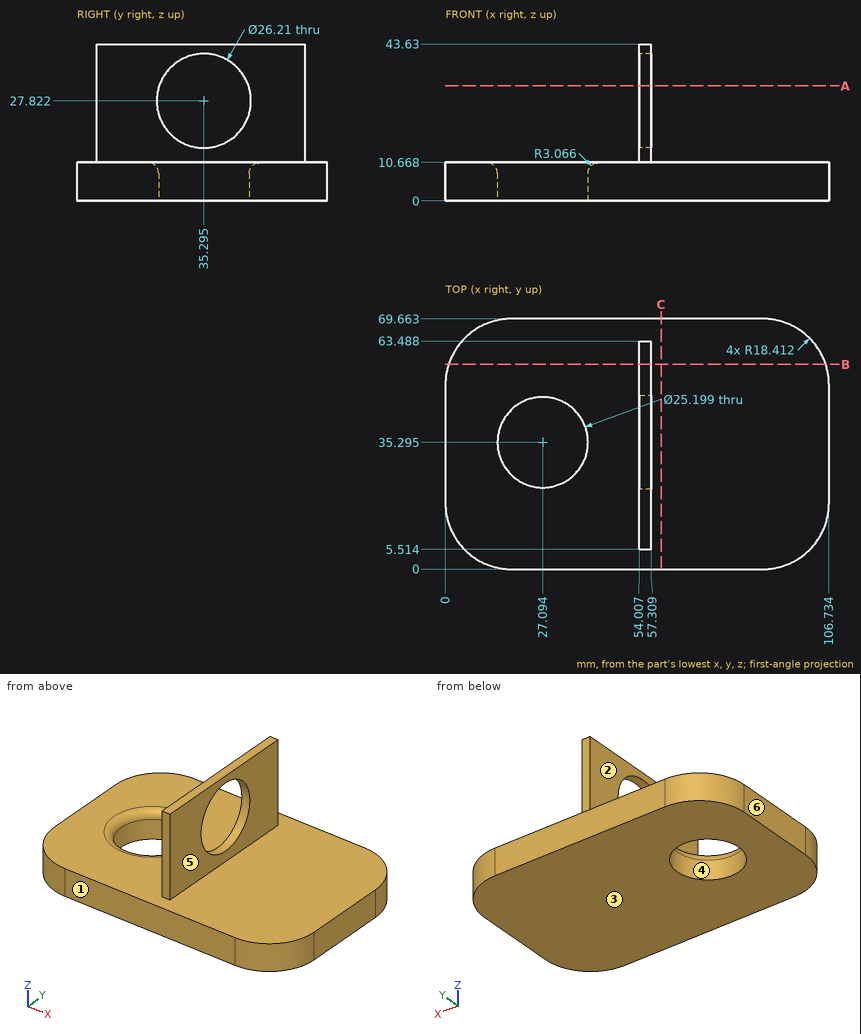
The figure shows three views and two pictorial views of one solid part (mm, origin at its lowest corner). Answer the questions. A direction names the side the tool comes from. Round coordinates to 2 decimals unless told otherwise and drop trailing zeros. Write each loop counter-clockwise with the first axis right and the second up, starting at its lowest first coordinate (ties: lowest second). Pieces come first, ordered by that corner, then holes. Notation, with made-up numbers: (-22.75, 2) - (10.25, 2) arc R17 ccw to (10.25, 20) - close; hole circle Ø2 at (21, 1). An arc over 180 degrees is marked (long way). Use one line per item in the form item = value. Start each with the question number.
Item 1: Determine the mould class of the marked faces 3, 4, 5 and 6 for opening direction X: +X half, -X half, draft (parallel to the pull), parting line (faces both ways), or undercut.
Item 2: Flat-ended cylindrical pins translate along their axes: pin 1 Ø1.7 at (x, z) = (56, 32) entering from -Y; pin 2 Ø8 at (x, y) = (17, 36) entering from +Z; pin 3 Ø6 at (x, z) = (56, 28) entering from +Y; pin 4 Ø1 at (x, z) = (27.5, 11) entering from +Y. Find the tip coordinate at first contact, or state that the pin passes through.
Item 3: A tool of negligible diameter and unlimited length cuts with its end or side. For the marked faces 1 and 2, from which of +Z, -Z, +X, -X, +Y, -Y can it reach the whole face along a straight path? Write none if from no direction.
Item 4: Find the intervals of material crossed by line 1 (Z direction, x = 16.5, y = 48); line 2 (X direction, y = 50, z = 30.5); line 3 (X direction, y = 30.5, z = 9.5) (1 decimal), in increasing order. Write a range as [from, to].
Item 5: A cutting plane is placed at B-B (y = 57). Write down the section's boundary in (x, z), plus the area to 3 significant figures.
Item 6: A cutting plane is placed at A-A (z = 32). Write down the section's boundary in (x, y) (1 decimal).
Item 7: A cutting plane is placed at C-C (x = 60). Write down the section's boundary in (y, z).
The answers:
q1.face_3 = draft
q1.face_4 = undercut
q1.face_5 = +X half
q1.face_6 = -X half
q2.pin_1 = 5.51
q2.pin_2 = 10.25
q2.pin_3 = 63.49
q2.pin_4 = 69.66
q3.face_1 = +Z, -Z, +X, -X, -Y
q3.face_2 = +Z, -X, +Y, -Y
q4.line_1 = [0, 10.67]
q4.line_2 = [54.01, 57.31]
q4.line_3 = [0, 14.7], [39.5, 106.7]
q5.outline = (0.92, 0) - (105.81, 0) - (105.81, 10.67) - (57.31, 10.67) - (57.31, 43.63) - (54.01, 43.63) - (54.01, 10.67) - (0.92, 10.67) - close
q5.area = 1,230 mm^2
q6.outline = (54, 5.5) - (57.3, 5.5) - (57.3, 22.9) - (54, 22.9) - close; (54, 47.7) - (57.3, 47.7) - (57.3, 63.5) - (54, 63.5) - close
q7.outline = (0, 0) - (69.66, 0) - (69.66, 10.67) - (0, 10.67) - close
